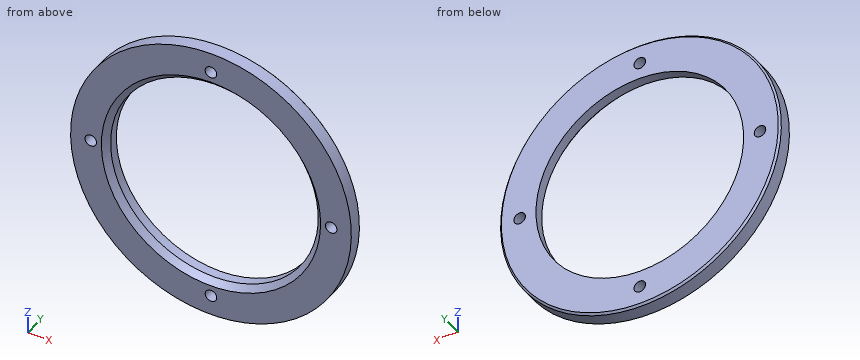
```python
from build123d import *

# Parameters (mm, degrees)
SKETCH_1_R          = 73
SKETCH_1_R_2        = 54
EXTRUDE_1_DEPTH     = 8
SKETCH_2_R          = 3
CUT_EXTRUDE_1_DEPTH = 10
CHAMFER_1_SIZE      = 1
CHAMFER_2_SIZE      = 3


with BuildPart() as part:
    # Эскиз1 → Бобышка-Вытянуть1 (new body)
    with BuildSketch(Plane(origin=(0, 0, 0), x_dir=(1, 0, 0), z_dir=(0, 1, 0))):
        with Locations(Location((0, 0, 0), (0, 0, 270))):
            Circle(SKETCH_1_R)
        with Locations(Location((0, 0, 0), (0, 0, 270))):
            Circle(SKETCH_1_R_2, mode=Mode.SUBTRACT)
    extrude(amount=EXTRUDE_1_DEPTH)

    # Эскиз2 → Вырез-Вытянуть1 (cut)
    with BuildSketch(Plane(origin=(0, 8, 0), x_dir=(-1, 0, 0), z_dir=(0, 1, 0))):
        with Locations(Location((62.5, 0, 0), (0, 0, 90))):
            Circle(SKETCH_2_R)
        with Locations(Location((0, -62.5, 0), (0, 0, 90))):
            Circle(SKETCH_2_R)
        with Locations(Location((0, 62.5, 0), (0, 0, 90))):
            Circle(SKETCH_2_R)
        with Locations(Location((-62.5, 0, 0), (0, 0, 90))):
            Circle(SKETCH_2_R)
    extrude(amount=-CUT_EXTRUDE_1_DEPTH, mode=Mode.SUBTRACT)

    # Фаска1
    chamfer_1_edges = [part.edges().sort_by_distance(p)[0] for p in [
        (0, 8, -73),
    ]]
    chamfer(chamfer_1_edges, length=CHAMFER_1_SIZE)

    # Фаска2
    chamfer_2_edges = [part.edges().sort_by_distance(p)[0] for p in [
        (0, 0, -54),
    ]]
    chamfer(chamfer_2_edges, length=CHAMFER_2_SIZE)


solid = part.part
```
The model under review builds one solid part; all positions refer to its coordinate system, in mm. Round coordinates to 2 decimals unless told otherwise and drop trailing zeros. Order: outer loops, then holes, each group sorted by start corner. A loop starts at its lowest first (then second) coordinate and runs counter-clockwise, first axis right, second up. Notation, with made-up numbers: (75, 49.5) - (102, 49.5) arc R11 ccw to (102, 60.5) - close; hole circle Ø3 at (88.5, 24). An arc over 180 degrees is marked (long way). Answer in a Markdown table with one row per item.
(1) Take a section at B-B on y = 1.5. Write out the cut boundary in (x, z), plus the area to 3 significant figures.
Result set:
| item | result |
|---|---|
| outline | circle Ø146 at (0, 0); hole circle Ø6 at (-62.5, 0); hole circle Ø111 at (0, 0); hole circle Ø6 at (0, -62.5); hole circle Ø6 at (0, 62.5); hole circle Ø6 at (62.5, 0) |
| area | 6,950 mm2 |
(2) For line 1 (X direction, y = 6.7, z = 0); line 2 (Z direction, x = 44, y = 5.75); line 3 (X direction, y = 5, z = 43), list the stretches that pass through material, from the lowest coordinate up. Write a range as from..to.
Result set:
| item | result |
|---|---|
| line 1 | x = -73..-65.5, -59.5..-54, 54..59.5, 65.5..73 |
| line 2 | z = -58.25..-31.3, 31.3..58.25 |
| line 3 | x = -58.99..-32.66, 32.66..58.99 |
(3) Clearance check with flat-ended pins moving along their axes: P1, Ø4, axis at x = -10.5, y = 1, coming from the +Z side; P2, Ø1.5, axis at y = 3, z = 20, coming from the +X side. State where each tip first meets the part, or that it passes through.
Result set:
| item | result |
|---|---|
| P1 | stops at z = 72.5 |
| P2 | stops at x = 70.42 |
(4) Take a section at A-A on x = 0. Write out the cut boundary in (y, z), plus the area to 3 significant figures.
Result set:
| item | result |
|---|---|
| outline | (0, -73) - (7, -73) - (8, -72) - (8, -65.5) - (0, -65.5) - close; (0, -59.5) - (8, -59.5) - (8, -54) - (3, -54) - (0, -57) - close; (0, 57) - (3, 54) - (8, 54) - (8, 59.5) - (0, 59.5) - close; (0, 65.5) - (8, 65.5) - (8, 72) - (7, 73) - (0, 73) - close |
| area | 198 mm2 |
